Verification items for this drawing (mm, ordinates from the low corner). A direction names the side the tool comes from. Round coordinates to 2 decimals unless told otherwise and drop trailing zeros. Order: outer loops, then holes, each group sorted by start corner. A loop starts at its lowest first (then second) coordinate and runs counter-clockwise, first axis right, second up. Notation, with made-up numbers: (-31.5, 26) -> (7.5, 26) arc R29 cw to (7.5, 46) -> close; hole circle Ø5 at (61, 1). An arc over 180 degrees is marked (long way). Put each result on its own line as item: value.
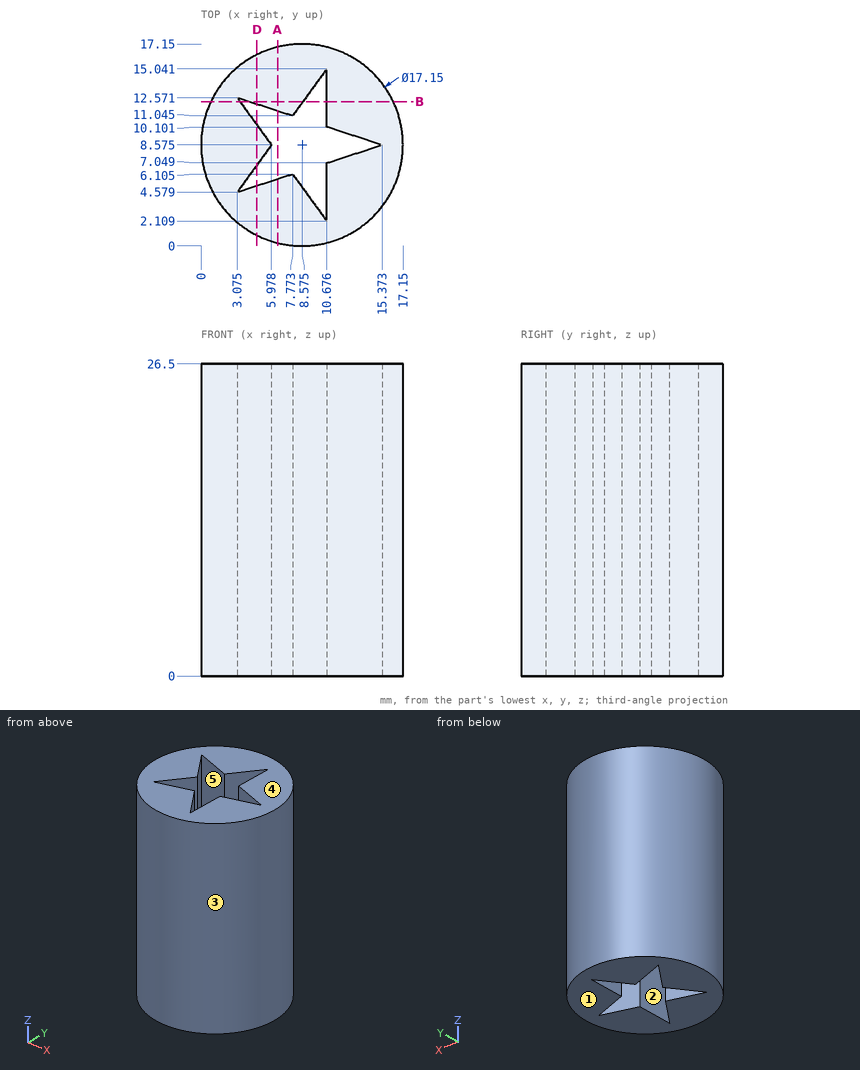
Item 1: Release check for a two-part mould opening along Y. For the marked faces 3, 4 and 5 record: +Y half, -Y half, draft (parallel to the pull), parting line (faces both ways), or undercut.
Check sheet entries:
face 3: parting line
face 4: draft
face 5: undercut
Item 2: Tool access check on the marked faces 1 and 2. Record the directions out of +Z, -Z, +X, -X, +Y, -Y that give a thin tool (end or side, any length) a straight path to the whole face; none if there is none.
Check sheet entries:
face 1: -Z, +X, -X, +Y, -Y
face 2: +Z, -Z
Item 3: Section check A-A on x = 6.5. Record the boundary of the cut face in (y, z) (1 decimal), then the cut area to 3 significant figures.
Check sheet entries:
outline: (0.3, 0) -> (5.7, 0) -> (5.7, 26.5) -> (0.3, 26.5) -> close; (11.5, 0) -> (16.9, 0) -> (16.9, 26.5) -> (11.5, 26.5) -> close
area: 288 mm^2
Item 4: Section check D-D on x = 4.75. State how many separate pieces and enclosed holes the cut face has.
Check sheet entries:
separate pieces: 3
enclosed holes: 0
Item 5: Material ranges on L1, parallel to Y at x = 4.25, z = 11.5 (1 decimal); L2, parallel to Y at x = 3.5, z = 2.25 (1 decimal); L3, parallel to Y at x = 15, z = 23.5 (1 decimal), recorded low to high. Write a range as [from, to].
Check sheet entries:
L1: y = [1.2, 5], [6.2, 11], [12.2, 16]
L2: y = [1.7, 4.7], [5.2, 12], [12.4, 15.5]
L3: y = [2.9, 8.5], [8.7, 14.3]
Item 6: Section check B-B on y = 12.25. Record the boundary of the cut face in (x, z) (1 decimal), then the cut area to 3 significant figures.
Check sheet entries:
outline: (0.8, 0) -> (3.3, 0) -> (3.3, 26.5) -> (0.8, 26.5) -> close; (4.1, 0) -> (8.6, 0) -> (8.6, 26.5) -> (4.1, 26.5) -> close; (10.7, 0) -> (16.3, 0) -> (16.3, 26.5) -> (10.7, 26.5) -> close
area: 337 mm^2
Item 7: Gauge pin test, flat ends, axial feed: pin 1 Ø1.5 at (y, z) = (13.5, 19.5) entering from -X (1 decimal); pin 2 Ø1 at (y, z) = (13, 5.5) entering from -X; pin 3 Ø1.5 at (y, z) = (11, 6.5) entering from -X (1 decimal). Record the tip position at first contact, or that the pin passes through.
Check sheet entries:
pin 1: stops at x = 1.1
pin 2: stops at x = 0.95
pin 3: stops at x = 0.2
